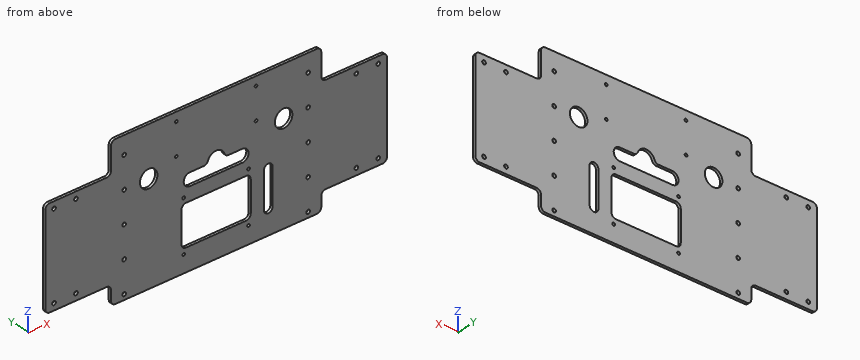
from build123d import *

# Parameters (mm, degrees)
SKETCH_1_W          = 240
SKETCH_1_H          = 166
EXTRUDE_1230_DEPTH  = 3
SKETCH_4_R          = 2.1
SKETCH_4_R_2        = 1.55
CUT_EXTRUDE_3_DEPTH = 251.068459046
SKETCH_5_R          = 1.55
SKETCH_5_R_2        = 10
SKETCH_5_W          = 79
SKETCH_5_H          = 45
CUT_EXTRUDE_4_DEPTH = 251.068459046
SKETCH_6_W          = 75
SKETCH_6_H          = 110
SKETCH_6_R          = 2.1
EXTRUDE_1_DEPTH     = 3
FILLET_1_R          = 5


with BuildPart() as part:
    # 草图1 → Extrude 1230 (new body)
    with BuildSketch(Plane(origin=(0, 0, 0), x_dir=(1, 0, 0), z_dir=(0, 1, 0))):
        with Locations((31.575924772, -115.871750732)):
            Rectangle(SKETCH_1_W, SKETCH_1_H)
    extrude(amount=EXTRUDE_1230_DEPTH)

    # 草图4 → 切除-拉伸3 (cut, through all)
    with BuildSketch(Plane(origin=(0, 3, 0), x_dir=(1, 0, 0), z_dir=(0, 1, 0))):
        with Locations(Location((-73.424075228, -73.871750732, 0), (0, 0, 270))):
            Circle(SKETCH_4_R)
        with Locations(Location((136.575924772, -178.871750732, 0), (0, 0, 90))):
            Circle(SKETCH_4_R)
        with Locations(Location((-73.424075228, -108.871750732, 0), (0, 0, 270))):
            Circle(SKETCH_4_R)
        with Locations(Location((-73.424075228, -143.871750732, 0), (0, 0, 270))):
            Circle(SKETCH_4_R)
        with Locations(Location((-73.424075228, -178.871750732, 0), (0, 0, 270))):
            Circle(SKETCH_4_R)
        with Locations(Location((136.575924772, -143.871750732, 0), (0, 0, 90))):
            Circle(SKETCH_4_R)
        with Locations(Location((136.575924772, -108.871750732, 0), (0, 0, 90))):
            Circle(SKETCH_4_R)
        with Locations(Location((136.575924772, -73.871750732, 0), (0, 0, 90))):
            Circle(SKETCH_4_R)
        with Locations(Location((-73.424075228, -38.871750732, 0), (0, 0, 270))):
            Circle(SKETCH_4_R)
        with Locations(Location((136.575924772, -38.871750732, 0), (0, 0, 90))):
            Circle(SKETCH_4_R)
        with Locations(Location((77.075924772, -188.871750732, 0), (0, 0, 270))):
            Circle(SKETCH_4_R_2)
        with Locations(Location((-13.924075228, -188.871750732, 0), (0, 0, 90))):
            Circle(SKETCH_4_R_2)
        with Locations(Location((77.075924772, -153.871750732, 0), (0, 0, 270))):
            Circle(SKETCH_4_R_2)
        with Locations(Location((-13.924075228, -153.871750732, 0), (0, 0, 90))):
            Circle(SKETCH_4_R_2)
    extrude(amount=-CUT_EXTRUDE_3_DEPTH, mode=Mode.SUBTRACT)

    # 草图5 → 切除-拉伸4 (cut, through all)
    with BuildSketch(Plane(origin=(0, 3, 0), x_dir=(1, 0, 0), z_dir=(0, 1, 0))):
        with Locations(Location((-5.424075228, -51.871750732, 0), (0, 0, 270))):
            Circle(SKETCH_5_R)
        with Locations(Location((68.575924772, -51.871750732, 0), (0, 0, 90))):
            Circle(SKETCH_5_R)
        with Locations(Location((68.575924772, -108.871750732, 0), (0, 0, 270))):
            Circle(SKETCH_5_R)
        with Locations(Location((-5.424075228, -108.871750732, 0), (0, 0, 90))):
            Circle(SKETCH_5_R)
        with Locations(Location((-45.424075228, -143.871750732, 0), (0, 0, 270))):
            Circle(SKETCH_5_R_2)
        with Locations(Location((108.575924772, -143.871750732, 0), (0, 0, 90))):
            Circle(SKETCH_5_R_2)
        with Locations((31.575924772, -80.371750732)):
            Rectangle(SKETCH_5_W, SKETCH_5_H)
        with BuildLine():
            Line((86.075924772, -100.371750732), (86.075924772, -60.371750732))
            ThreePointArc((86.075924772, -60.371750732), (91.075924772, -55.371750732), (96.075924772, -60.371750732))
            Line((96.075924772, -60.371750732), (96.075924772, -100.371750732))
            ThreePointArc((96.075924772, -100.371750732), (91.075924772, -105.371750732), (86.075924772, -100.371750732))
        make_face()
        with BuildLine():
            Line((1.575924772, -117.871750732), (61.575924772, -117.871750732))
            ThreePointArc((61.575924772, -117.871750732), (68.575924772, -124.871750732), (61.575924772, -131.871750732))
            Line((61.575924772, -131.871750732), (41.575924772, -131.871750732))
            ThreePointArc((41.575924772, -131.871750732), (31.575924772, -141.871750732), (21.575924772, -131.871750732))
            Line((21.575924772, -131.871750732), (1.575924772, -131.871750732))
            ThreePointArc((1.575924772, -131.871750732), (-5.424075228, -124.871750732), (1.575924772, -117.871750732))
        make_face()
    extrude(amount=-CUT_EXTRUDE_4_DEPTH, mode=Mode.SUBTRACT)

    # 草图6 → 凸台-拉伸1 (add)
    # profile 1 of 2: a face of its own
    with BuildSketch(Plane(origin=(0, 0, 0), x_dir=(1, 0, 0), z_dir=(0, 1, 0))):
        with Locations((-125.924075228, -108.871750732)):
            Rectangle(SKETCH_6_W, SKETCH_6_H)
        with Locations(Location((-153.424075228, -61.371750732, 0), (0, 0, 270))):
            Circle(SKETCH_6_R, mode=Mode.SUBTRACT)
        with Locations(Location((-153.424075228, -156.371750732, 0), (0, 0, 90))):
            Circle(SKETCH_6_R, mode=Mode.SUBTRACT)
        with Locations(Location((-128.424075228, -61.371750732, 0), (0, 0, 270))):
            Circle(SKETCH_6_R, mode=Mode.SUBTRACT)
        with Locations(Location((-128.424075228, -156.371750732, 0), (0, 0, 90))):
            Circle(SKETCH_6_R, mode=Mode.SUBTRACT)
    # profile 2 of 2: a face of its own
    with BuildSketch(Plane(origin=(0, 0, 0), x_dir=(1, 0, 0), z_dir=(0, 1, 0))):
        with Locations((189.075924772, -108.871750732)):
            Rectangle(SKETCH_6_W, SKETCH_6_H)
        with Locations(Location((216.575924772, -156.371750732, 0), (0, 0, 270))):
            Circle(SKETCH_6_R, mode=Mode.SUBTRACT)
        with Locations(Location((216.575924772, -61.371750732, 0), (0, 0, 90))):
            Circle(SKETCH_6_R, mode=Mode.SUBTRACT)
        with Locations(Location((191.575924772, -156.371750732, 0), (0, 0, 270))):
            Circle(SKETCH_6_R, mode=Mode.SUBTRACT)
        with Locations(Location((191.575924772, -61.371750732, 0), (0, 0, 90))):
            Circle(SKETCH_6_R, mode=Mode.SUBTRACT)
    extrude(amount=EXTRUDE_1_DEPTH)

    # 圆角1
    fillet_1_edges = [part.edges().sort_by_distance(p)[0] for p in [
        (41.575924772, 1.5, 131.871750732),
        (21.575924772, 1.5, 131.871750732),
        (-7.924075228, 1.5, 102.871750732),
        (-7.924075228, 1.5, 57.871750732),
        (71.075924772, 1.5, 57.871750732),
        (71.075924772, 1.5, 102.871750732),
        (-88.424075228, 1.5, 163.871750732),
        (-88.424075228, 1.5, 53.871750732),
        (-163.424075228, 1.5, 53.871750732),
        (-163.424075228, 1.5, 163.871750732),
        (226.575924772, 1.5, 53.871750732),
        (151.575924772, 1.5, 53.871750732),
        (151.575924772, 1.5, 163.871750732),
        (226.575924772, 1.5, 163.871750732),
        (-88.424075228, 1.5, 198.871750732),
        (-88.424075228, 1.5, 32.871750732),
        (151.575924772, 1.5, 32.871750732),
        (151.575924772, 1.5, 198.871750732),
    ]]
    fillet(fillet_1_edges, radius=FILLET_1_R)


solid = part.part
Geometry: final body of the model. Coordinates: model frame, mm. Give positions to 0.01 mm unless a question says otherwise; leave off trailing zeros. Write each loop counter-clockwise with the first axis right and the second up, starting at its lowest first coordinate (ties: lowest second). Pieces come first, ordered by that corner, then holes.
(1) Ray query, line 1 (X direction, y = 1.9, z = 91); line 2 (X direction, y = 1.05, z = 98.5); line 3 (Z direction, x = 138, y = 0.55). Return the intervals inside material, ascending.
(2) Cut plane B-B, the plane z = 125.5. Return loops of the section in (x, y), then the cut area to 3 significant figures.
(3) First-contact query: P1, Ø2.5, axis at x = 136.58, z = 38.87, coming from the -Y side. Flat tip, straight axial feed; report the tip coordinate or a pass-through.
(4) Cut plane A-A, the plane x = 55. Return loops of the section in (y, z), then the cut area to 3 significant figures.
(5) Cut plane C-C, the plane y = 2.5. Give the number of separate pieces and of enclosed holes in the cut face, then the cut area to 3 significant figures.
Values follow:
1. line 1: x = -163.42 to -7.92, 71.08 to 86.08, 96.08 to 226.58
1. line 2: x = -163.42 to -7.88, 71.04 to 86.08, 96.08 to 226.58
1. line 3: z = 32.87 to 37.33, 40.42 to 72.33, 75.42 to 107.33, 110.42 to 142.33, 145.42 to 177.33, 180.42 to 198.87
2. outline: (-163.42, 0) - (-5.4, 0) - (-5.4, 3) - (-163.42, 3) - close; (68.55, 0) - (226.58, 0) - (226.58, 3) - (68.55, 3) - close
2. area: 948 mm2
3. P1: passes through
4. outline: (0, 32.87) - (3, 32.87) - (3, 57.87) - (0, 57.87) - close; (0, 102.87) - (3, 102.87) - (3, 117.87) - (0, 117.87) - close; (0, 131.87) - (3, 131.87) - (3, 198.87) - (0, 198.87) - close
4. area: 321 mm2
5. separate pieces: 1
5. enclosed holes: 31
5. area: 50,200 mm2
